Can you work these out from the model? Positions are in its coordinate system, mm. Face numbers are marked on the shaded views. A direction names the side the tool comes from. Give positions to 0.01 mm unless a question says otherwise; leave off trailing zeros. Loops run counter-clockwise (first coordinate to the right, second up) from the corner with the lowest first, then second, coordinate; pieces in that order, holes last.
from build123d import *

# Parameters (mm, degrees)
SKETCH1_R           = 25.4
BOSS_EXTRUDE1_DEPTH = 8.255
FILLET1_R           = 2.54
SKETCH3_R           = 3.2258
CUT_EXTRUDE1_DEPTH  = 40.533531954
SKETCH4_R           = 13.335
SKETCH4_R_2         = 9.652
CUT_EXTRUDE2_DEPTH  = 6.604


# Read off the part's stored shape, not the designer's step: Cut-Revolve-Thin6
with BuildPart() as part:
    # Sketch1 → Boss-Extrude1 (new, symmetric)
    with BuildSketch(Plane.XY):
        Circle(SKETCH1_R)
    extrude(amount=BOSS_EXTRUDE1_DEPTH, both=True)

    # Cut-Revolve-Thin6 outline → Cut-Revolve-Thin6 (revolve, cut)
    with BuildSketch(Plane.XZ):
        Polygon((25.4, 8.255), (22.903425716, 8.255), (25.4, 1.395718529), align=None)
        Polygon((25.4, -8.255), (25.4, -1.395718529), (22.903425716, -8.255), align=None)
    revolve(axis=Axis((0, 0, 0), (0, 0, 1)), mode=Mode.SUBTRACT)

    # Fillet1
    fillet1_edges = [part.edges().sort_by_distance(p)[0] for p in [
        (-25.4, 0, -1.395718529),
        (-25.4, 0, 1.395718529),
    ]]
    fillet(fillet1_edges, radius=FILLET1_R)

    # Sketch3 → Cut-Extrude1 (cut, through all)
    with BuildSketch(Plane.XY.offset(8.255)):
        Circle(SKETCH3_R)
    extrude(amount=-CUT_EXTRUDE1_DEPTH, mode=Mode.SUBTRACT)

    # Sketch4 → Cut-Extrude2 (cut)
    with BuildSketch(Plane.XY.offset(8.255)):
        Circle(SKETCH4_R)
        Circle(SKETCH4_R_2, mode=Mode.SUBTRACT)
    cut_extrude2 = extrude(amount=-CUT_EXTRUDE2_DEPTH, mode=Mode.SUBTRACT)

    # Mirror1: Cut-Extrude2 across plane
    add(cut_extrude2.mirror(Plane.XY), mode=Mode.SUBTRACT)


solid = part.part
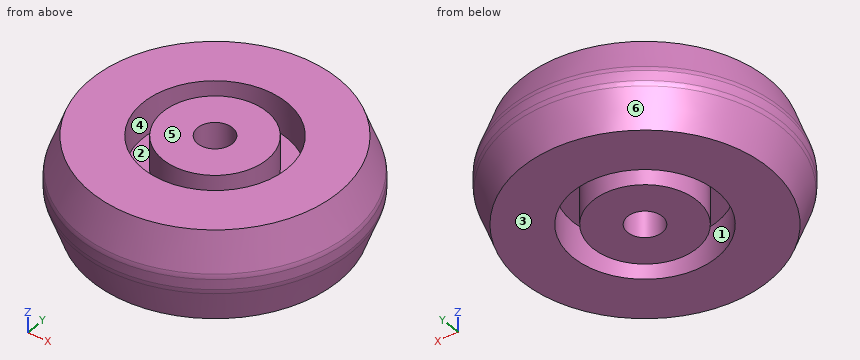
(1) Suppose I cut it at B-B on z = -5.25. List the corners of the cut face in (x, y) for me (3 decimals), plus the area to 3 significant figures.
Returned:
outline: circle Ø47.994 at (0, 0); circle Ø19.304 at (0, 0); hole circle Ø26.67 at (0, 0); hole circle Ø6.452 at (0, 0)
area: 1,510 mm2
(2) Thinking about a two-plate mould opening in Y: for the marked faces 4, 5 and 6, which applies, pulls with the +Y half, pulls with the -Y half, needs draft (parallel to the pull), parting line crosses it, or undercut?
Returned:
face 4: undercut
face 5: needs draft
face 6: parting line crosses it
(3) Will these pins go through, and if not, where does the flat tip stop? P1, Ø8, axis at y = 10.5, z = -5, coming from the -X side; P2, Ø2, axis at y = 18, z = 0, coming from the -X side; P3, Ø1, axis at x = -19.5, z = -2, coming from the -Y side.
Returned:
P1: stops at x = -23.92
P2: stops at x = -18.87
P3: stops at y = -16.59
(4) Which directions (+Z, -Z, +X, -X, +Y, -Y) give clear straight access to the entire face, cutting with the end or side of a thin tool? Please do the marked faces 1, 2 and 3.
Returned:
face 1: -Z
face 2: +Z
face 3: -Z, +X, -X, +Y, -Y
(5) Please list where these lines run through material, in increasing order: probe 1 along Y at (x, z) = (0, -5.5) (3 decimals); probe 2 along X at (y, z) = (4, 7); probe 3 along Y at (x, z) = (0, 6.5) (3 decimals).
Returned:
probe 1: y = -23.906 to -13.335, -9.652 to -3.226, 3.226 to 9.652, 13.335 to 23.906
probe 2: x = -23.02 to -12.72, -8.78 to 8.78, 12.72 to 23.02
probe 3: y = -23.542 to -13.335, -9.652 to -3.226, 3.226 to 9.652, 13.335 to 23.542
(6) Suppose I cut it at A-A on z = 4. List the corners of the cut face in (x, y) for me (3 decimals), plus the area to 3 significant figures.
Returned:
outline: circle Ø48.904 at (0, 0); circle Ø19.304 at (0, 0); hole circle Ø26.67 at (0, 0); hole circle Ø6.452 at (0, 0)
area: 1,580 mm2
